Here's the drawing with two shaded views (mm, measured from the low corner). I have some questions. Round coordinates to 2 decimals unless told otherwise and drop trailing zeros. Loops run counter-clockwise (first coordinate to the right, second up) from the corner with the lowest first, then second, coordinate; pieces in that order, holes last.
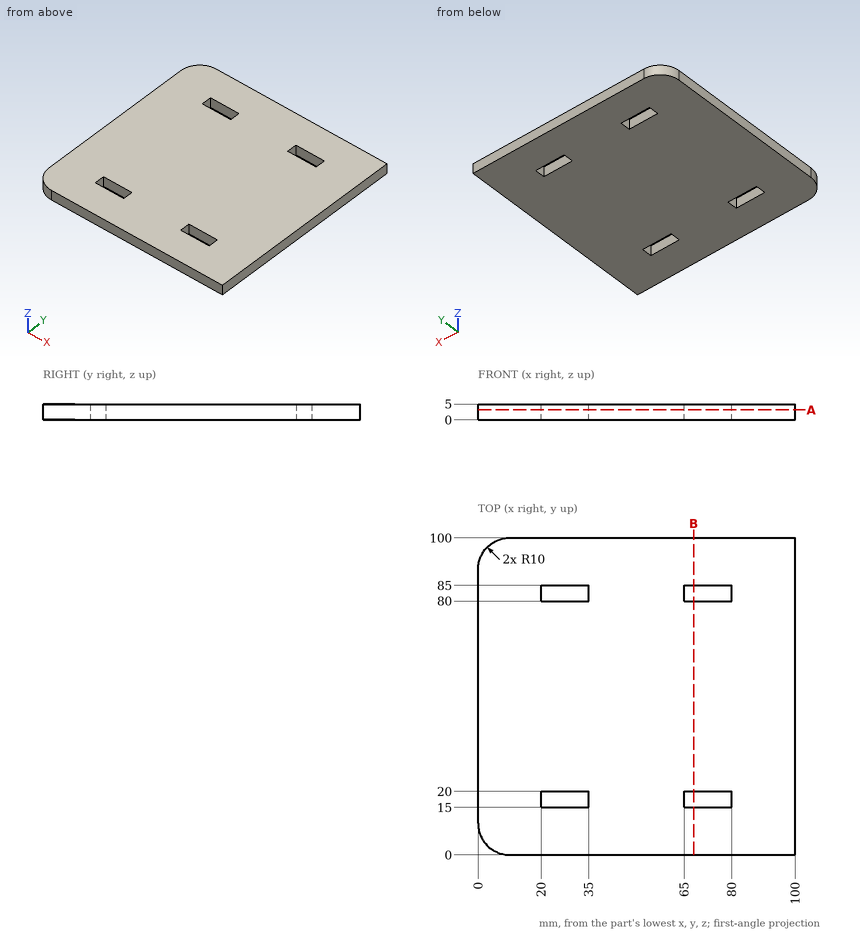
(1) If we section it at B-B, the plane x = 68: List the corners of the cut face in (y, z) for me.
Worked answers:
outline: (0, 0) - (15, 0) - (15, 5) - (0, 5) - close; (20, 0) - (80, 0) - (80, 5) - (20, 5) - close; (85, 0) - (100, 0) - (100, 5) - (85, 5) - close
(2) If I drill on line 1 (X direction, y = 19, z = 0.7); line 2 (Y direction, x = 77, z = 4.25); line 3 (X direction, y = 8, z = 1.55), over which ranges is the centre line in solid material (lowest first)?
Worked answers:
line 1: x = 0 to 20, 35 to 65, 80 to 100
line 2: y = 0 to 15, 20 to 80, 85 to 100
line 3: x = 0.2 to 100
(3) If we section it at A-A, the plane z = 3.15: List the corners of the cut face in (x, y) for me.
Worked answers:
outline: (0, 10) arc R10 ccw to (10, 0) - (100, 0) - (100, 100) - (10, 100) arc R10 ccw to (0, 90) - close; hole (20, 15) - (35, 15) - (35, 20) - (20, 20) - close; hole (20, 80) - (35, 80) - (35, 85) - (20, 85) - close; hole (65, 15) - (80, 15) - (80, 20) - (65, 20) - close; hole (65, 80) - (80, 80) - (80, 85) - (65, 85) - close
